Check sheet for the modelled part. Datum: model origin and axes. Units: mm. A direction names the side the tool comes from. Round coordinates to 2 decimals unless told otherwise and drop trailing zeros. Order: outer loops, then holes, each group sorted by start corner. A loop starts at its lowest first (then second) coordinate and runs counter-clockwise, first axis right, second up.
(1) Thickness scan on probe 1 along Z at (x, y) = (-23.8, 1); probe 2 along X at (y, z) = (0.9, -25.1); probe 3 along Y at (x, z) = (-3.75, -15.25). Record the ranges inside material, lowest first.
(2) Sectioned sample at A-A, the plane x = -23.8. Enter the section's corners in (y, z), and give its area (3 significant figures).
(3) Sectioned sample at D-D, the plane x = -18. Enter the section's corners in (y, z), and give its area (3 significant figures).
(4) Mould release check, pull along X, two halves, no side actions. Record for faces 1 (the cylindrical face through (-9.148, 3.062, -19.951)), 2 (the cylindrical face through (-23.225, 1.183, -23.714)), 3 (the flat face through (-16.4, 6, -20)): released by +X, released by -X, zero draft, split by the parting line, or undercut.
(5) Sectioned sample at C-C, the plane z = -13. Enter the section's corners in (x, y).
(6) Tool access check on faces 4 (the cylindrical face through (-13.3, 2.9, -12.3)), 5 (the flat face through (-10.4, 6, -20)), 6 (the flat face through (-22.5, 2.4, -3.6)). Record the directions out of +Z, -Z, +X, -X, +Y, -Y that give a thin tool (end or side, any length) a straight path to the whole face; none if there is none.
(7) Depth check by flat-ended pin: pin 1 (1.8 mm diameter, centred on x = -3, z = -26, fed in from +Y); pin 2 (3 mm diameter, centred on x = -20, z = -23.5, fed in from +Y); pin 3 (5 mm diameter, centred on x = -23.5, z = -3.5, fed in from +Y); pin 4 (2.5 mm diameter, centred on x = -23.8, z = -4.9, fed in from -Y). Enter the tip coordinate at first touch or a pass-through.
Autodesk Inventor part; units mm, degrees
ref_plane "YZ Plane" through (0, 0, 0) normal (1, 0, 0) x (0, 1, 0)
ref_plane "XZ Plane" through (0, 0, 0) normal (0, 1, 0) x (-1, 0, 0)
ref_plane "XY Plane" through (0, 0, 0) normal (0, 0, 1) x (1, 0, 0)
sketch "Sketch1" plane through (0, 0, 0) normal (0, 1, 0) x (-1, 0, 0)
  line L0 (0, 0) -> (30, 0)
  line L1 (30, 0) -> (30, -30)
  line L2 (30, -30) -> (0, -30)
  line L3 (0, -30) -> (0, 0)
  dimension "d0" = 30
  dimension "d1" = 30
extrude "Extrusion1" add sketch "Sketch1" along normal blind 2.5
sketch "Sketch2" plane through (0, 2.5, 0) normal (0, 1, 0) x (1, 0, 0)
  line L0 (-30, 0) -> (0, 0)
  line L1 (0, 0) -> (0, 30)
  line L2 (0, 30) -> (-30, 30)
  point P0 (-3, 4.9)
  point P1 (-3, 25.1)
  point P2 (-23.8, 25.1)
  point P3 (-23.8, 4.9)
  dimension "d14" = 20.2
  dimension "d15" = 20.8
  dimension "d16" = 4.9
  dimension "d17" = 20.2
  dimension "d18" = 3
  dimension "d19" = 20.8
  dimension "d20" = 4.9
  dimension "d21" = 4.9
hole "Hole1" at (-3, 2.5, -4.9) at (-3, 2.5, -25.1) at (-23.8, 2.5, -25.1) at (-23.8, 2.5, -4.9) direction (0, -1, 0) diameter 3 end through all counterbore diameter 6 counterbore depth 0.1
sketch "Sketch3" plane through (0, 2.5, 0) normal (0, 1, 0) x (1, 0, 0)
  line L0 (-30, 30) -> (-30, 0)
  circle A0 centre (-30, 15) radius 1
  point P0 (0, 0)
  point P1 (-30, 16)
  point P2 (-30, 14)
  dimension "d11" = 2
extrude "Extrusion2" cut sketch "Sketch3" against normal blind 1 contours A0 L0 picked at (-29.6652, 15.1995)
sketch "Sketch4" plane through (0, 2.5, 0) normal (0, 1, 0) x (1, 0, 0)
  line L0 (-10.4, 11.5) -> (-16.4, 11.5)
  line L1 (-16.4, 11.5) -> (-16.4, 8.5)
  line L2 (-16.4, 8.5) -> (-10.4, 8.5)
  line L3 (-10.4, 8.5) -> (-10.4, 11.5)
  line L4 (-30, 0) -> (0, 0)
  line L5 (0, 0) -> (0, 30)
  line L6 (-10.4, 18.5) -> (-16.4, 18.5)
  line L7 (-16.4, 18.5) -> (-16.4, 21.5)
  line L8 (-16.4, 21.5) -> (-10.4, 21.5)
  line L9 (-10.4, 21.5) -> (-10.4, 18.5)
  line L10 (-30, 30) -> (-30, 16)
  dimension "d22" = 6
  dimension "d23" = 3
  dimension "d24" = 8.5
  dimension "d25" = 10.4
  dimension "d26" = 3
  dimension "d27" = 7
  dimension "d28" = 13.6
  dimension "d29" = 10.4
extrude "Extrusion3" add sketch "Sketch4" along normal blind 7
fillet "Fillet1" radius 3 8 edges at (-10.4, 9.5, -10) (-16.4, 9.5, -10) (-16.4, 9.5, -20) (-10.4, 9.5, -20) (-10.4, 2.5, -20) (-10.4, 2.5, -10) (-16.4, 2.5, -20) (-16.4, 2.5, -10)
sketch "Sketch5" plane through (-7.4, 2.5, -11.5) normal (0, 0, -1) x (-1, 0, 0)
  circle A0 centre (6, 4.5) radius 1.5
  line L0 (12, 0) -> (0, 0)
  line L1 (3, 3) -> (3, 4)
  point P0 (-7.4, -2.5)
  dimension "d33" = 3
  dimension "d34" = 4.5
  dimension "d35" = 3
extrude "Extrusion4" add sketch "Sketch5" along normal up to surface (7 mm away)
fillet "Fillet2" radius 1 2 edges at (-11.9, 7, -11.5) (-11.9, 7, -18.5)
fillet "Fillet3" radius 2 4 edges at (-13.4, 2.5, -11.5) (-13.4, 2.5, -18.5) (-13.4, 2.5, -8.5) (-13.4, 2.5, -21.5)
sketch "Sketch6" plane through (0, 2.5, 0) normal (0, 1, 0) x (1, 0, 0)
  point P0 (0, 0)
properties part number "Upper mount"
Derived:
1. probe 1: z = -30 to -26.6, -23.6 to -6.4, -3.4 to 0
1. probe 2: x = -30 to -25.3, -22.3 to -4.5, -1.5 to 0
1. probe 3: y = 0 to 2.5
2. outline: (0, -30) - (2.5, -30) - (2.5, -28.1) - (2.4, -28.1) - (2.4, -26.6) - (0, -26.6) - close; (0, -23.6) - (2.4, -23.6) - (2.4, -22.1) - (2.5, -22.1) - (2.5, -7.9) - (2.4, -7.9) - (2.4, -6.4) - (0, -6.4) - close; (0, -3.4) - (2.4, -3.4) - (2.4, -1.9) - (2.5, -1.9) - (2.5, 0) - (0, 0) - close
2. area: 59.4 mm2
3. outline: (0, -30) - (2.5, -30) - (2.5, -23.5) arc R2 cw to (2.85, -22.37) - (2.85, -17.63) arc R2 cw to (2.5, -16.5) - (2.5, -13.5) arc R2 cw to (2.85, -12.37) - (2.85, -7.63) arc R2 cw to (2.5, -6.5) - (2.5, 0) - (0, 0) - close
3. area: 78.8 mm2
4. face 1: released by +X
4. face 2: undercut
4. face 3: released by -X
5. outline: (-30, 0) - (0, 0) - (0, 2.5) - (-7.4, 2.5) arc R3 cw to (-8.01, 2.56) - (-18.79, 2.56) arc R3 cw to (-19.4, 2.5) - (-30, 2.5) - close; circle Ø3 at (-13.4, 7)
6. face 4: +X, -X
6. face 5: +Z, -Z, +X, +Y
6. face 6: +Y
7. pin 1: stops at y = 2.4
7. pin 2: stops at y = 2.6
7. pin 3: stops at y = 2.5
7. pin 4: passes through
